Geometry check sheet. Reference: the model listing, model coordinates, mm. A direction names the side the tool comes from. Give positions to 0.01 mm unless a question says otherwise; leave off trailing zeros. Loops run counter-clockwise (first coordinate to the right, second up) from the corner with the lowest first, then second, coordinate; pieces in that order, holes last. Notation, with made-up numbers: (59.25, -6.75) -> (103.25, -6.75) arc R12 ccw to (103.25, 11.25) -> close; hole circle Ø10 at (-37.5, 84). An arc over 180 degrees is marked (long way). Write item = value, one per line.
```python
from build123d import *

# Parameters (mm, degrees)
SKETCH1_W            = 54
SKETCH1_H            = 77
BOSS_EXTRUDE1_DEPTH  = 5
SKETCH2_R            = 2.55
CUT_EXTRUDE1_DEPTH   = 48.289005065
LPATTERN1_COUNT      = 2
LPATTERN1_PITCH      = 42
LPATTERN1_COUNT_DIR2 = 2
LPATTERN1_PITCH_DIR2 = 63
SKETCH3_W            = 30
SKETCH3_H            = 50
CUT_EXTRUDE2_DEPTH   = 48.289005065
FILLET1_R            = 5


with BuildPart() as part:
    # Sketch1 → Boss-Extrude1 (new body)
    with BuildSketch(Plane(origin=(0, 0, 0), x_dir=(1, 0, 0), z_dir=(0, 1, 0))):
        Rectangle(SKETCH1_W, SKETCH1_H)
    extrude(amount=BOSS_EXTRUDE1_DEPTH)

    # Sketch2 → Cut-Extrude1 (cut, through all)
    with BuildSketch(Plane(origin=(0, 5, 0), x_dir=(1, 0, 0), z_dir=(0, 1, 0))):
        with Locations(Location((-21, 31.5, 0), (0, 0, 270))):
            Circle(SKETCH2_R)
    cut_extrude1 = extrude(amount=-CUT_EXTRUDE1_DEPTH, mode=Mode.SUBTRACT)

    # LPattern1: Cut-Extrude1 2 × 2
    with Locations(*[(i * LPATTERN1_PITCH, 0, j * LPATTERN1_PITCH_DIR2) for i in range(LPATTERN1_COUNT) for j in range(LPATTERN1_COUNT_DIR2) if (i, j) != (0, 0)]):
        add(cut_extrude1, mode=Mode.SUBTRACT)

    # Sketch3 → Cut-Extrude2 (cut, through all)
    with BuildSketch(Plane(origin=(0, 5, 0), x_dir=(1, 0, 0), z_dir=(0, 1, 0))):
        Rectangle(SKETCH3_W, SKETCH3_H)
    extrude(amount=-CUT_EXTRUDE2_DEPTH, mode=Mode.SUBTRACT)

    # Fillet1
    fillet1_edges = [part.edges().sort_by_distance(p)[0] for p in [
        (15, 2.5, -25),
        (15, 2.5, 25),
        (-15, 2.5, 25),
        (-15, 2.5, -25),
        (27, 2.5, 38.5),
        (-27, 2.5, 38.5),
        (-27, 2.5, -38.5),
        (27, 2.5, -38.5),
    ]]
    fillet(fillet1_edges, radius=FILLET1_R)


solid = part.part
```
Item 1: Gauge pin test, flat ends, axial feed: pin 1 (8 mm diameter, centred on x = -13.5, z = -11, fed in from +Y); pin 2 (2 mm diameter, centred on x = -13.5, z = -14.5, fed in from -Y). Record the tip position at first contact, or that the pin passes through.
Answer:
pin_1 = 5
pin_2 = through
Item 2: Section check A-A, the plane z = 11. Record the cut outline in (x, y).
Answer:
outline = (-27, 0) -> (-15, 0) -> (-15, 5) -> (-27, 5) -> close; (15, 0) -> (27, 0) -> (27, 5) -> (15, 5) -> close
Item 3: Thickness scan on L1, parallel to X at y = 2.15, z = 31.5; L2, parallel to Z at x = 3, y = 1.55; L3, parallel to X at y = 1.9, z = 20. Record the ranges inside material, lowest first. Write a range as [from, to].
Answer:
L1 = [-27, -23.55], [-18.45, 18.45], [23.55, 27]
L2 = [-38.5, -25], [25, 38.5]
L3 = [-27, -15], [15, 27]
Item 4: Tool access check on faces 1 (the flat face through (-15, 3, 0)), 2 (the cylindrical face through (-25.57, 2.54, -37)). Record the directions out of +Z, -Z, +X, -X, +Y, -Y that give a thin tool (end or side, any length) a straight path to the whole face; none if there is none.
Answer:
face_1 = +Y, -Y
face_2 = -Z, -X, +Y, -Y
Item 5: Section check B-B, the plane x = 21. Record the cut outline in (y, z).
Answer:
outline = (0, -38.5) -> (5, -38.5) -> (5, -34.05) -> (0, -34.05) -> close; (0, -28.95) -> (5, -28.95) -> (5, 28.95) -> (0, 28.95) -> close; (0, 34.05) -> (5, 34.05) -> (5, 38.5) -> (0, 38.5) -> close
Item 6: Draft check along X on faces 3 (the flat face through (18, 5, -1)), 4 (the cylindrical face through (14, 2, -23)), 5 (the cylindrical face through (25.5, 2.54, 37.07)). Enter one of: +X half, -X half, draft (parallel to the pull), parting line (faces both ways), or undercut.
Answer:
face_3 = draft
face_4 = undercut
face_5 = +X half
Item 7: Section check C-C, the plane z = 31.5. Record the cut outline in (x, y), plus the area to 3 significant figures.
Answer:
outline = (-27, 0) -> (-23.55, 0) -> (-23.55, 5) -> (-27, 5) -> close; (-18.45, 0) -> (18.45, 0) -> (18.45, 5) -> (-18.45, 5) -> close; (23.55, 0) -> (27, 0) -> (27, 5) -> (23.55, 5) -> close
area = 219 mm^2
Item 8: Section check D-D, the plane x = 2. Record the cut outline in (y, z).
Answer:
outline = (0, -38.5) -> (5, -38.5) -> (5, -25) -> (0, -25) -> close; (0, 25) -> (5, 25) -> (5, 38.5) -> (0, 38.5) -> close
